Verification items for the finished model (mm, model axes). Face numbers are marked on the shaded views. A direction names the side the tool comes from. Coordinates: 2 decimals unless noted, no trailing zeros. Order: outer loops, then holes, each group sorted by start corner. A loop starts at its lowest first (then second) coordinate and runs counter-clockwise, first axis right, second up.
Q1. Cross-section at A-A, the plane z = 19. Record the boundary of the cut face in (x, y), and give its area (3 significant figures).
Q2. Set-up check for the marked faces 1 and 2: record each of +Z, -Z, +X, -X, +Y, -Y from which the full face is reachable in a straight line by a thin tool's end or side.
Q3. Depth check by flat-ended pin: P1, Ø10, axis at y = -0.5, z = 20.5, coming from the +X side; P2, Ø1.5, axis at x = -1, y = 0, coming from the +Z side; P3, Ø1, axis at x = -5, y = 14, coming from the +Z side. Enter the tip coordinate at first touch or a pass-through.
Q4. Thickness scan on line 1 (Y direction, x = -4, z = 12.5); line 2 (Y direction, x = 0, z = -5); line 3 (Z direction, x = -6, y = -2.5). Record the ranges inside material, lowest first.
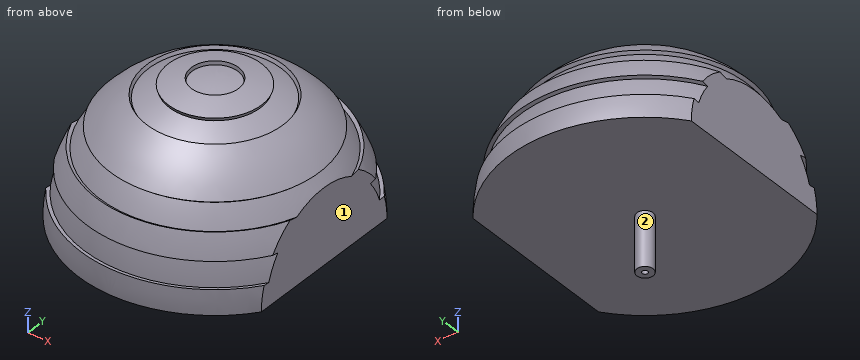
from build123d import *

# Parameters (mm, degrees)
REVOLVE_1_ANGLE     = 180
CUT_EXTRUDE_1_DEPTH = 44.56107781
SHELL_1_T           = -5
SKETCH_3_R          = 1.5
SKETCH_3_R_2        = 0.5
EXTRUDE_3_DEPTH     = 5
EXTRUDE_START       = 10
SKETCH_5_R          = 1.5
SKETCH_5_R_2        = 0.5
EXTRUDE_4_DEPTH     = 10


with BuildPart() as part:
    # 草图1 → 旋转1 (revolve)
    with BuildSketch(Plane.XY):
        with BuildLine():
            Line((0, 25.15), (0, -25.15))
            ThreePointArc((0, -25.15), (25.15, 0), (0, 25.15))
        make_face()
    revolve(axis=Axis((0, 25.15, 0), (0, -1, 0)), revolution_arc=REVOLVE_1_ANGLE)

    # 草图2 → 切除-拉伸1 (cut, through all)
    with BuildSketch(Plane(origin=(0, 0, 0), x_dir=(-1, 0, 0), z_dir=(0, 0, -1))):
        with BuildLine():
            ThreePointArc((25.15, 0), (23.877083587, 7.899834137), (20.18718653, 15))
            Line((20.18718653, 15), (20.18718653, -15))
            ThreePointArc((20.18718653, -15), (23.877083587, -7.899834137), (25.15, 0))
        make_face()
        with BuildLine():
            Line((-20.18718653, -15), (-20.18718653, 15))
            ThreePointArc((-20.18718653, 15), (-25.15, 0), (-20.18718653, -15))
        make_face()
    extrude(amount=-CUT_EXTRUDE_1_DEPTH, mode=Mode.SUBTRACT)

    # 抽壳1
    shell_1_openings = [part.faces().sort_by_distance(p)[0] for p in [
        (0, 0, 0),
    ]]
    offset(amount=SHELL_1_T, openings=shell_1_openings)

    # 草图3 → 凸台-拉伸3 (add)
    # profile 1 of 2: a face of its own
    with BuildSketch(Plane(origin=(0, 0, 0), x_dir=(-1, 0, 0), z_dir=(0, 0, -1))):
        with BuildLine():
            ThreePointArc((-15.18718653, 13.242804284), (0, 20.15), (15.18718653, 13.242804284))
            Line((15.18718653, 13.242804284), (15.18718653, -13.242804284))
            ThreePointArc((15.18718653, -13.242804284), (0, -20.15), (-15.18718653, -13.242804284))
            Line((-15.18718653, -13.242804284), (-15.18718653, 13.242804284))
        make_face()
        Circle(SKETCH_3_R, mode=Mode.SUBTRACT)
    # profile 2 of 2: a face of its own
    with BuildSketch(Plane(origin=(0, 0, 0), x_dir=(-1, 0, 0), z_dir=(0, 0, -1))):
        Circle(SKETCH_3_R)
        Circle(SKETCH_3_R_2, mode=Mode.SUBTRACT)
    extrude(amount=-EXTRUDE_3_DEPTH)

    # 草图5 → 凸台-拉伸4 (add)
    with BuildSketch(Plane(origin=(0, 0, 0), x_dir=(-1, 0, 0), z_dir=(0, 0, -1)).offset(EXTRUDE_START)):
        Circle(SKETCH_5_R)
        Circle(SKETCH_5_R_2, mode=Mode.SUBTRACT)
    extrude(amount=-EXTRUDE_4_DEPTH)

    # 草图6 → 切除-旋转2 (revolve, cut)
    with BuildSketch(Plane(origin=(0, 0, 0), x_dir=(0, 0, -1), z_dir=(1, 0, 0))):
        with BuildLine():
            ThreePointArc((-8.379493511, 23.022469209), (-6.341066605, 23.665182744), (-4.254380353, 24.127789949))
            Line((-4.254380353, 24.127789949), (-4.367251668, 24.767914988))
            ThreePointArc((-4.367251668, 24.767914988), (-6.509298984, 24.293034531), (-8.601806605, 23.633269413))
            Line((-8.601806605, 23.633269413), (-8.379493511, 23.022469209))
        make_face()
        with BuildLine():
            ThreePointArc((-15.748296437, 18.768088856), (-14.052622691, 20.069225085), (-12.25, 21.217622393))
            Line((-12.25, 21.217622393), (-12.575, 21.780538905))
            ThreePointArc((-12.575, 21.780538905), (-14.425447374, 20.601673914), (-16.166108384, 19.266017744))
            Line((-16.166108384, 19.266017744), (-15.748296437, 18.768088856))
        make_face()
        with BuildLine():
            ThreePointArc((-23.022469209, 8.379493511), (-22.204540782, 10.354147413), (-21.217622393, 12.25))
            Line((-21.217622393, 12.25), (-21.780538905, 12.575))
            ThreePointArc((-21.780538905, 12.575), (-22.793640844, 10.628849283), (-23.633269413, 8.601806605))
            Line((-23.633269413, 8.601806605), (-23.022469209, 8.379493511))
        make_face()
        with BuildLine():
            Line((-25.15, 0), (-24.5, 0))
            ThreePointArc((-24.5, 0), (-24.406770103, 2.135315697), (-24.127789949, 4.254380353))
            Line((-24.127789949, 4.254380353), (-24.767914988, 4.367251668))
            ThreePointArc((-24.767914988, 4.367251668), (-25.054296657, 2.19196693), (-25.15, 0))
        make_face()
    revolve(axis=Axis((0, 0, 0), (0, 0, 1)), mode=Mode.SUBTRACT)


solid = part.part
Check values:
1. outline: circle Ø32.96 at (0, 0); hole circle Ø13.42 at (0, 0)
1. area: 712 mm2
2. face 1: +Z, -Z, +X, +Y, -Y
2. face 2: -Z
3. P1: stops at x = 19.27
3. P2: stops at z = 24.5
3. P3: stops at z = 20.64
4. line 1: y = -21.45 to -21.28, -20.69 to -15.29, 15.29 to 20.69, 21.28 to 21.45
4. line 2: y = -1.5 to -0.5, 0.5 to 1.5
4. line 3: z = 0 to 5, 19.07 to 24.3
